The model under review builds one solid part; all positions refer to its coordinate system, in mm. Face numbers are marked on the shaded views. A direction names the side the tool comes from. Give positions to 0.01 mm unless a question says otherwise; leave off trailing zeros. Loops run counter-clockwise (first coordinate to the right, second up) from the corner with the lowest first, then second, coordinate; pieces in that order, holes last. Notation, with made-up numbers: (-33, 79.5) - (-3, 79.5) arc R32 ccw to (-3, 114.5) - close; hole circle Ø3 at (67, 89.5). An arc over 180 degrees is marked (long way). Return JSON: item names as keys, results as strings. Group by question number.
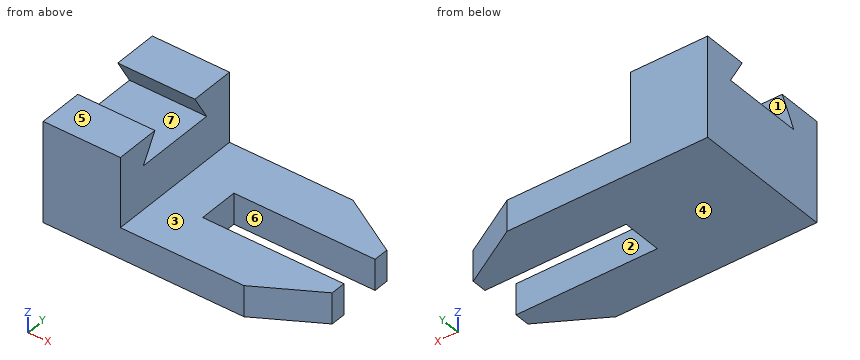
```python
from build123d import *

# Parameters (mm, degrees)
F1_DEPTH = 70
F3_DEPTH = 38.3278513458
F4_W     = 70.1527081109
F4_H     = 20
F5_DEPTH = 15.3706480632
F8_DEPTH = 15.3706480632


with BuildPart() as f1:
    # F0 (on Front) → F1 (new body)
    with BuildSketch(Plane.XZ):
        Polygon((-13.0350217989, 34.6303519368), (-51.3618731447, 34.6303519368), (-51.3618731447, -15.3696480632), (78.6381268553, -15.3696480632), (78.6381268553, 0), (-13.0350217989, 0), align=None)
    extrude(amount=F1_DEPTH)

    # F2 (on face) → F3 (cut, through all)
    with BuildSketch(Plane.YZ.offset(-13.0350217989)):
        Polygon((-22.1706290543, 34.6303519368), (-47.8293709457, 34.6303519368), (-55.3293709457, 21.6399708801), (-35, 21.6399708801), (-14.6706290543, 21.6399708801), align=None)
    extrude(amount=-F3_DEPTH, mode=Mode.SUBTRACT)

    # F4 (on face) → F5 (cut, through all)
    with BuildSketch(Plane.XY):
        with Locations((43.5617727999, -35)):
            Rectangle(F4_W, F4_H)
    extrude(amount=-F5_DEPTH, mode=Mode.SUBTRACT)

    # F7 (on face) → F8 (cut, through all)
    with BuildSketch(Plane.XY):
        Polygon((78.6381268553, -52.5), (48.3272377229, -70), (78.6381268553, -70), align=None)
        Polygon((48.3272377229, 0), (78.6381268553, -17.5), (78.6381268553, 0), align=None)
    extrude(amount=-F8_DEPTH, mode=Mode.SUBTRACT)


solid = f1.part
```
1) We need section C-C, the plane z = 26. Write out the cut boundary in (x, y).
2) For pin 1 Ø21 at (x, y) = (25, -25.5) entering from +Z; pin 2 Ø17.5 at (y, z) = (-44.5, 21.5) entering from +X (3 decimals), all flat-tipped, find the tip position at first contact; note any pin that passes through.
3) We need section D-D, the plane x = -36.5. Write out the cut boundary in (y, z), plus the area to 3 significant figures.
4) We need section B-B, the plane z = -11.5. Write out the cut boundary in (x, y), plus the area to 3 significant figures.
5) Draft analysis for pull direction Z (two halves, no side actions). For the marked faces 4, 5, 6 and 7, state which applies: +Z half, -Z half, draft (parallel to the pull), parting line (faces both ways), or undercut.
6) To check wall thickness, follow line 1 (Y direction, x = 10, z = -1); line 2 (X direction, y = -36.5, z = -7); line 3 (Z direction, x = 46, y = -65). State the ranges of each line that lie inside material, in increasing order.
7) We need section A-A, the plane x = 33.5. Write out the cut boundary in (y, z), plus the area to 3 significant figures.
8) Tool access review of the marked faces 1, 2 and 3: name each direction out of +Z, -Z, +X, -X, +Y, -Y from which nothing blocks a thin tool from reaching the whole face with its end or side.
Findings:
{
 "1": {"outline": "(-51.36, -70) - (-13.04, -70) - (-13.04, -52.81) - (-51.36, -52.81) - close; (-51.36, -17.19) - (-13.04, -17.19) - (-13.04, 0) - (-51.36, 0) - close"},
 "2": {"pin 1": "stops at z = 0", "pin 2": "stops at x = -13.035"},
 "3": {"outline": "(-70, -15.37) - (0, -15.37) - (0, 34.63) - (-22.17, 34.63) - (-14.67, 21.64) - (-55.33, 21.64) - (-47.83, 34.63) - (-70, 34.63) - close", "area": "3,070 mm^2"},
 "4": {"outline": "(-51.36, -70) - (48.33, -70) - (78.64, -52.5) - (78.64, -45) - (8.49, -45) - (8.49, -25) - (78.64, -25) - (78.64, -17.5) - (48.33, 0) - (-51.36, 0) - close", "area": "7,170 mm^2"},
 "5": {"face 4": "-Z half", "face 5": "+Z half", "face 6": "draft", "face 7": "undercut"},
 "6": {"line 1": "y = -70 to -45, -25 to 0", "line 2": "x = -51.36 to 8.49", "line 3": "z = -15.37 to 0"},
 "7": {"outline": "(-70, -15.37) - (-45, -15.37) - (-45, 0) - (-70, 0) - close; (-25, -15.37) - (0, -15.37) - (0, 0) - (-25, 0) - close", "area": "768 mm^2"},
 "8": {"face 1": "+X, -X", "face 2": "+Z, -Z, +X", "face 3": "+Z, +X, +Y, -Y"}
}
